```python
from build123d import *

# Parameters (mm, degrees)
SKETCH3_W           = 20
SKETCH3_H           = 40
BOSS_EXTRUDE2_DEPTH = 20
FILLET2_R           = 7.5
SKETCH4_R           = 3.175
CUT_EXTRUDE2_DEPTH  = 21
SKETCH5_W           = 20
SKETCH5_H           = 17.5
CUT_EXTRUDE3_DEPTH  = 20
CUT_EXTRUDE4_REACH  = 24.5
SKETCH6_R           = 3.175
SKETCH7_R           = 6.35
CUT_EXTRUDE5_DEPTH  = 41


with BuildPart() as part:
    # Sketch3 → Boss-Extrude2 (new body, symmetric)
    with BuildSketch(Plane(origin=(0, 0, 0), x_dir=(1, 0, 0), z_dir=(0, 1, 0))):
        Rectangle(SKETCH3_W, SKETCH3_H)
    extrude(amount=BOSS_EXTRUDE2_DEPTH, both=True)

    # Fillet2
    fillet2_edges = [part.edges().sort_by_distance(p)[0] for p in [
        (0, 20, -20),
    ]]
    fillet(fillet2_edges, radius=FILLET2_R)

    # Sketch4 → Cut-Extrude2 (cut, through all)
    with BuildSketch(Plane.ZY.offset(10)):
        with Locations((-12.5, 12.5)):
            Circle(SKETCH4_R)
    extrude(amount=-CUT_EXTRUDE2_DEPTH, mode=Mode.SUBTRACT)

    # Sketch5 → Cut-Extrude3 (cut)
    with BuildSketch(Plane(origin=(0, 20, 0), x_dir=(1, 0, 0), z_dir=(0, 1, 0))):
        with Locations((0, -11.25)):
            Rectangle(SKETCH5_W, SKETCH5_H)
    extrude(amount=-CUT_EXTRUDE3_DEPTH, mode=Mode.SUBTRACT)

    # Sketch6 → Cut-Extrude4 (cut, up to next)
    with BuildSketch(Plane.XY.offset(2.5), mode=Mode.PRIVATE) as cut_extrude4_sk1:
        with Locations((0, 12.5)):
            Circle(SKETCH6_R)
    cut_extrude4_tool1 = extrude(cut_extrude4_sk1.sketch, amount=-CUT_EXTRUDE4_REACH, mode=Mode.PRIVATE) & part.part
    add(cut_extrude4_tool1.solids().sort_by_distance((0, 12.5, 2.5))[0], mode=Mode.SUBTRACT)

    # Sketch7 → Cut-Extrude5 (cut, through all)
    with BuildSketch(Plane.XY.offset(20)):
        with Locations((0, -10)):
            Circle(SKETCH7_R)
    extrude(amount=-CUT_EXTRUDE5_DEPTH, mode=Mode.SUBTRACT)


solid = part.part
```
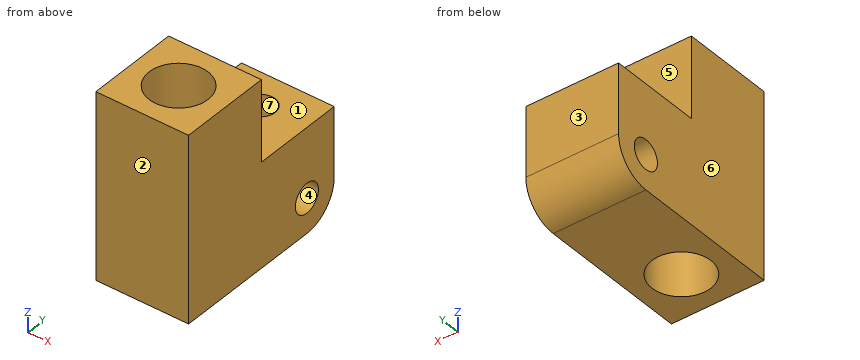
Model file for the job. Use its own axes, mm. Face numbers are marked on the shaded views. A direction names the side the tool comes from. Round coordinates to 2 decimals unless told otherwise and drop trailing zeros. Write each loop counter-clockwise with the first axis right and the second up, starting at its lowest first coordinate (ties: lowest second). Pieces come first, ordered by that corner, then holes. Notation, with made-up numbers: (-29, 79) -> (-4, 79) arc R14 cw to (-4, 100) -> close; hole circle Ø4 at (15.5, -9.75). An arc over 180 degrees is marked (long way). Answer as CSV lines item,"result".
1. Pin check, flat tips, straight feed: pin 1 Ø5 at (x, z) = (1, 10.5) entering from +Y; pin 2 Ø7.5 at (x, y) = (0, 12.5) entering from +Z. Stop position of each tip, or through.
Resolved:
pin 1,"y = 0"
pin 2,"z = 2.5"
2. Drill centre lines: line 1 (Y direction, x = 0, z = 1.5) (3 decimals); line 2 (X direction, y = 12.5, z = -7.5) (3 decimals); line 3 (Z direction, x = -8, y = 2.5). Where is each one in solid material? Low to high.
Resolved:
line 1,"-20 to -16.35, -3.65 to 9.325, 15.675 to 20"
line 2,"-10 to -3.175, 3.175 to 10"
line 3,"-20 to 2.5"
3. Slice it at C-C, the plane x = 0. List the corners of the cut face in (y, z) (3 decimals).
Resolved:
outline,"(-20, -20) -> (-16.35, -20) -> (-16.35, 20) -> (-20, 20) -> close; (-3.65, -20) -> (12.5, -20) arc R7.5 ccw to (20, -12.5) -> (20, 2.5) -> (15.675, 2.5) -> (15.675, -12.5) arc R3.175 cw to (9.325, -12.5) -> (9.325, 2.5) -> (0, 2.5) -> (0, 20) -> (-3.65, 20) -> close"
4. Tool access for the marked faces 5, 6 and 7: list every direction of +Z, -Z, +X, -X, +Y, -Y with a clear straight run to the whole face (end or side of a thin tool).
Resolved:
face 5,"+Z, +X, -X, +Y"
face 6,"+Z, -Z, -X, +Y, -Y"
face 7,"+Z"
5. Mould opens along Y. For the marked faces 1, 2, 3 and 4 say: +Y half, -Y half, draft (parallel to the pull), parting line (faces both ways), or undercut.
Resolved:
face 1,"draft"
face 2,"-Y half"
face 3,"+Y half"
face 4,"undercut"
6. Slice it at B-B, the plane y = -10. List the corners of the cut face in (x, z).
Resolved:
outline,"(-10, -20) -> (-6.35, -20) -> (-6.35, 20) -> (-10, 20) -> close; (6.35, -20) -> (10, -20) -> (10, 20) -> (6.35, 20) -> close"
7. Slice it at D-D, the plane z = 11. List the corners of the cut face in (x, y), plus the area to 3 significant figures.
Resolved:
outline,"(-10, -20) -> (10, -20) -> (10, 0) -> (-10, 0) -> close; hole circle Ø12.7 at (0, -10)"
area,"273 mm²"
8. Slice it at A-A, the plane x = 4.75. List the corners of the cut face in (y, z) (3 decimals).
Resolved:
outline,"(-20, -20) -> (-14.214, -20) -> (-14.214, 20) -> (-20, 20) -> close; (-5.786, -20) -> (12.5, -20) arc R7.5 ccw to (20, -12.5) -> (20, 2.5) -> (0, 2.5) -> (0, 20) -> (-5.786, 20) -> close; hole circle Ø6.35 at (12.5, -12.5)"
